Verification items for the finished model (mm, model axes). Give positions to 0.01 mm unless a question says otherwise; leave off trailing zeros. Loops run counter-clockwise (first coordinate to the right, second up) from the corner with the lowest first, then second, coordinate; pieces in that order, holes last. Notation, with made-up numbers: (-3.5, 50) - (33.5, 50) arc R5 ccw to (33.5, 54) - close; hole circle Ø4 at (-27, 65.5). An arc over 180 degrees is marked (long way). Answer in a Markdown table with one row per item.
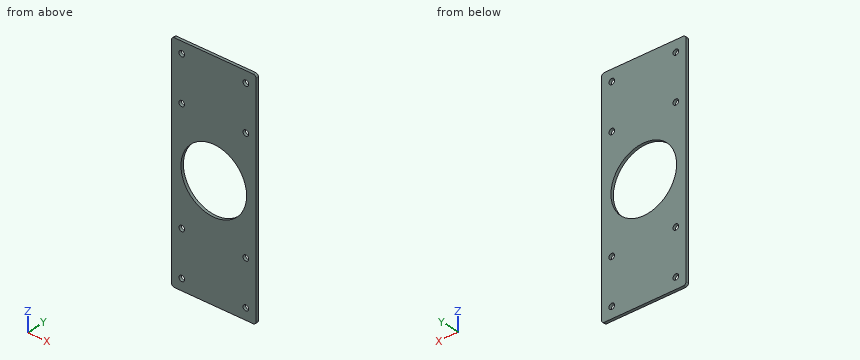
```python
from build123d import *

# Parameters (mm, degrees)
SKETCH1_W           = 90
SKETCH1_H           = 240
SKETCH1_R           = 35
SKETCH1_R_2         = 3
BOSS_EXTRUDE1_DEPTH = 3
FILLET1_R           = 3


with BuildPart() as part:
    # Sketch1 → Boss-Extrude1 (new body)
    with BuildSketch(Plane(origin=(0, 0, 0), x_dir=(1, 0, 0), z_dir=(0, 1, 0))):
        Rectangle(SKETCH1_W, SKETCH1_H)
        Circle(SKETCH1_R, mode=Mode.SUBTRACT)
        with Locations((-34.15, 60)):
            Circle(SKETCH1_R_2, mode=Mode.SUBTRACT)
        with Locations((34.15, 60)):
            Circle(SKETCH1_R_2, mode=Mode.SUBTRACT)
        with Locations((34.15, -60)):
            Circle(SKETCH1_R_2, mode=Mode.SUBTRACT)
        with Locations((-34.15, -60)):
            Circle(SKETCH1_R_2, mode=Mode.SUBTRACT)
        with Locations((-34.15, 108)):
            Circle(SKETCH1_R_2, mode=Mode.SUBTRACT)
        with Locations((34.15, 108)):
            Circle(SKETCH1_R_2, mode=Mode.SUBTRACT)
        with Locations((-34.15, -108)):
            Circle(SKETCH1_R_2, mode=Mode.SUBTRACT)
        with Locations((34.15, -108)):
            Circle(SKETCH1_R_2, mode=Mode.SUBTRACT)
    extrude(amount=BOSS_EXTRUDE1_DEPTH)

    # Fillet1
    fillet1_edges = [part.edges().sort_by_distance(p)[0] for p in [
        (45, 1.5, 120),
        (-45, 1.5, 120),
        (-45, 1.5, -120),
        (45, 1.5, -120),
    ]]
    fillet(fillet1_edges, radius=FILLET1_R)


solid = part.part
```
Q1. Sectioned sample at A-A (z = -108). Record the cut outline in (x, y).
Completed:
| item | result |
|---|---|
| outline | (-45, 0) - (-37.15, 0) - (-37.15, 3) - (-45, 3) - close; (-31.15, 0) - (31.15, 0) - (31.15, 3) - (-31.15, 3) - close; (37.15, 0) - (45, 0) - (45, 3) - (37.15, 3) - close |
Q2. Sectioned sample at D-D (z = 0). Record the cut outline in (x, y).
Completed:
| item | result |
|---|---|
| outline | (-45, 0) - (-35, 0) - (-35, 3) - (-45, 3) - close; (35, 0) - (45, 0) - (45, 3) - (35, 3) - close |
Q3. Sectioned sample at B-B (x = -3). Record the cut outline in (y, z), and give its area (3 significant figures).
Completed:
| item | result |
|---|---|
| outline | (0, -120) - (3, -120) - (3, -34.87) - (0, -34.87) - close; (0, 34.87) - (3, 34.87) - (3, 120) - (0, 120) - close |
| area | 511 mm^2 |
Q4. Sectioned sample at C-C (y = 2.25). Give the number of separate pieces and of enclosed holes in the cut face, and give its area (3 significant figures).
Completed:
| item | result |
|---|---|
| separate pieces | 1 |
| enclosed holes | 9 |
| area | 17,500 mm^2 |
Q5. Go/stop test with flat-tipped pins: P1, Ø3.5, axis at x = -34.15, z = 108, coming from the -Y side; P2, Ø8, axis at x = -34.15, z = -60, coming from the +Y side. Record where each tip stops, or that it passes through.
Completed:
| item | result |
|---|---|
| P1 | through |
| P2 | y = 3 |
Q6. Thickness scan on line 1 (X direction, y = 1.25, z = -60); line 2 (X direction, y = 1.4, z = 0); line 3 (Z direction, x = 1.5, y = 1.9). Record the ranges inside material, lowest first.
Completed:
| item | result |
|---|---|
| line 1 | -45 to -37.15, -31.15 to 31.15, 37.15 to 45 |
| line 2 | -45 to -35, 35 to 45 |
| line 3 | -120 to -34.97, 34.97 to 120 |
